```python
from build123d import *

# Parameters (mm, degrees)
F0_R     = 1
F0_R_2   = 3
F1_DEPTH = 1


with BuildPart() as f1:
    # F0 (on Front) → F1 (new body, symmetric)
    with BuildSketch(Plane.XZ):
        Polygon((-15, 0), (0, 0), (15, 0), (15, 5), (5, 27), (0, 27), (-5, 27), (-15, 5), align=None)
        with Locations((-12.7, 2.5)):
            Circle(F0_R, mode=Mode.SUBTRACT)
        with Locations((12.7, 2.5)):
            Circle(F0_R, mode=Mode.SUBTRACT)
        with Locations((0, 22)):
            Circle(F0_R_2, mode=Mode.SUBTRACT)
    extrude(amount=F1_DEPTH, both=True)


solid = f1.part
```
Input: part model. Units: mm. Frame: model coordinates. Coordinates: 2 decimals unless noted, no trailing zeros. Loops run counter-clockwise (first coordinate to the right, second up) from the corner with the lowest first, then second, coordinate; pieces in that order, holes last. Notation, with made-up numbers: M -26.5,77.5 L 10.5,77.5 A21 cw 10.5,100.5 Z; hole C 71,80.25 d5. An arc over 180 degrees is marked long. Use a Markdown table: item, result. Add a question column.
1) Draft query along Z for faces 1 (the cylindrical face through (-0.65, 0.01, 19.07)), 2 (the flat face through (0, 0, 0)), 3 (the flat face through (10, 0, 16)). Return one class per face: +Z half, -Z half, draft (parallel to the pull), parting line (faces both ways), or undercut.
2) Section B-B, the plane x = 0. Return the cut outline in (y, z).
3) Section C-C, the plane y = 0.4. Return the cut outline in (x, z).
4) Pin query (flat end, axial travel): P1, Ø1, axis at y = -0.5, z = 19, coming from the -X side. Return the tip coordinate at first contact, or that it passes through.
5) Section A-A, the plane z = 2.5. Return the cut outline in (x, y), plus the area to 3 significant figures.
6) Line query: L1, parallel to Z at x = 0, y = -0.3; L2, parallel to Z at x = 13.25, y = 0.85; L3, parallel to X at y = 0.55, z = 11. Output: solid intervals per line, ascending. Write a range as from..to.
7) Section D-D, the plane z = 22. Return the cut outline in (x, y), plus the area to 3 significant figures.
Answer below:
| question | item | result |
|---|---|---|
| 1 | face 1 | undercut |
| 1 | face 2 | -Z half |
| 1 | face 3 | +Z half |
| 2 | outline | M -1,0 L 1,0 L 1,19 L -1,19 Z; M -1,25 L 1,25 L 1,27 L -1,27 Z |
| 3 | outline | M -15,0 L 15,0 L 15,5 L 5,27 L -5,27 L -15,5 Z; hole C -12.7,2.5 d2; hole C 0,22 d6; hole C 12.7,2.5 d2 |
| 4 | P1 | x = -8.86 |
| 5 | outline | M -15,-1 L -13.7,-1 L -13.7,1 L -15,1 Z; M -11.7,-1 L 11.7,-1 L 11.7,1 L -11.7,1 Z; M 13.7,-1 L 15,-1 L 15,1 L 13.7,1 Z |
| 5 | area | 52.0 mm2 |
| 6 | L1 | 0..19, 25..27 |
| 6 | L2 | 0..1.66, 3.34..8.85 |
| 6 | L3 | -12.27..12.27 |
| 7 | outline | M -7.27,-1 L -3,-1 L -3,1 L -7.27,1 Z; M 3,-1 L 7.27,-1 L 7.27,1 L 3,1 Z |
| 7 | area | 17.1 mm2 |
